Here's how the part is built. I have some questions about the finished solid (model axes, mm). A direction names the side the tool comes from. Coordinates: 2 decimals unless noted, no trailing zeros. Write each loop counter-clockwise with the first axis right and the second up, starting at its lowest first coordinate (ties: lowest second). Pieces come first, ordered by that corner, then holes.
Item 1: For faces 5 (the face through (-1.588, 200, -13)), 6 (the face through (-14.08, -18.9, -24.6)), which set-ups out of +Z, -Z, +X, -X, +Y, -Y let a thin tool reach every point of the face, with its end or its side?
Item 2: If I drill on line 1 (Y direction, x = -12.7, z = -24.8); line 2 (Z direction, x = -16.75, y = 74), over which ranges is the centre line in solid material (lowest first)?
Item 3: If we section it at A-A (z = -19.5): Please give me the cut outline in (x, y), then the cut area to 3 significant figures.
Item 4: We'd pull the mould along Y, two halves only. Please class faces 1 (the face through (-13.5, 412.7, -0.8)), 2 (the face through (-14.08, -18.9, -0.78)), 3 (the face through (-13, 200, -1.588)), 4 (the face through (-24, -25.4, -13)): +Y half, -Y half, draft (parallel to the pull), parting line (faces both ways), or undercut.
Item 5: If we section it at B-B (y = 230.5): Please give me the cut outline in (x, z).
Item 6: If we section it at C-C (x = -12.7): Count the separate pieces of the cut face and the enclosed holes in it, then the cut area to 3 significant figures.
Autodesk Inventor part; units mm, degrees
ref_plane "YZ Plane" through (0, 0, 0) normal (1, 0, 0) x (0, 1, 0)
ref_plane "XZ Plane" through (0, 0, 0) normal (0, 1, 0) x (-1, 0, 0)
ref_plane "XY Plane" through (0, 0, 0) normal (0, 0, 1) x (1, 0, 0)
sketch "Sketch1" plane through (0, 0, 0) normal (0, 1, 0) x (-1, 0, 0)
  line L0 (0, 0) -> (25.4, 0)
  line L1 (25.4, 0) -> (25.4, -25.4)
  line L2 (25.4, -25.4) -> (0, -25.4)
  line L3 (0, -25.4) -> (0, 0)
  line L4 (23.8125, -23.8125) -> (23.8125, -1.5875)
  line L5 (23.8125, -1.5875) -> (1.5875, -1.5875)
  line L6 (1.5875, -1.5875) -> (1.5875, -23.8125)
  line L7 (1.5875, -23.8125) -> (23.8125, -23.8125)
  dimension "d0" = 25.4
  dimension "d1" = 25.4
  dimension "d2" = 1.5875
extrude "Extrusion1" add sketch "Sketch1" along normal blind 419.1
sketch "Sketch3" plane through (-25.4, 0, 0) normal (0, 0, 1) x (1, 0, 0)
  point P0 (25.4, 0)
sketch "Sketch4" plane through (-25.4, 0, 0) normal (0, 0, 1) x (1, 0, 0)
  circle A0 centre (12.7, 406.4) radius 6.35
  line L0 (25.4, 0) -> (0, 0)
  line L1 (25.4, 0) -> (25.4, 419.1)
  line L2 (1.5875, 419.1) -> (23.8125, 419.1)
  dimension "d8" = 12.7
  dimension "d28" = 12.7
  dimension "d29" = 12.7
extrude "Extrusion3" cut sketch "Sketch4" against normal blind 25.4
sketch "Sketch5" plane through (-25.4, 0, 0) normal (0, 0, 1) x (1, 0, 0)
  circle A0 centre (12.7, 266.7) radius 6.35
  line L0 (25.4, 0) -> (0, 0)
  dimension "d12" = 12.7
  dimension "d15" = 266.7
extrude "Extrusion4" cut sketch "Sketch5" against normal blind 25.4
sketch "Sketch7" plane through (0, 0, 0) normal (0, -1, 0) x (1, 0, 0)
  line L0 (0, 0) -> (-25.4, 0)
  line L1 (-25.4, 0) -> (-25.4, -25.4)
  line L2 (-25.4, -25.4) -> (0, -25.4)
  line L3 (0, -25.4) -> (0, 0)
  line L4 (-1.5875, -23.8125) -> (-23.8125, -23.8125)
  line L5 (-23.8125, -1.5875) -> (-1.5875, -1.5875)
  line L6 (-23.8125, -23.8125) -> (-1.5875, -23.8125)
  line L7 (-1.5875, -23.8125) -> (-1.5875, -1.5875)
  line L8 (-1.5875, -1.5875) -> (-23.8125, -1.5875)
  line L9 (-23.8125, -1.5875) -> (-23.8125, -23.8125)
extrude "Extrusion6" add sketch "Sketch7" along normal blind 25.4
sketch "Sketch8" plane through (-25.4, 419.1, 0) normal (0, 0, 1) x (1, 0, 0)
  circle A0 centre (12.7, -431.8) radius 6.35
  line L0 (25.4, -444.5) -> (25.4, 0)
  line L1 (25.4, -444.5) -> (0, -444.5)
  point P0 (25.4, -419.1)
  dimension "d23" = 12.7
  dimension "d24" = 12.7
  dimension "d27" = 12.7
extrude "Extrusion7" cut sketch "Sketch8" against normal blind 25.4
properties part number "AP 2"
Answer list:
1. face 5: +Y, -Y
1. face 6: +Z, -Z
2. line 1: y = -25.4 to -19.05, -6.35 to 260.35, 273.05 to 400.05, 412.75 to 419.1
2. line 2: z = -25.4 to -23.81, -1.59 to 0
3. outline: (-25.4, -25.4) - (-23.81, -25.4) - (-23.81, 419.1) - (-25.4, 419.1) - close; (-1.59, -25.4) - (0, -25.4) - (0, 419.1) - (-1.59, 419.1) - close
3. area: 1,410 mm2
4. face 1: undercut
4. face 2: undercut
4. face 3: draft
4. face 4: -Y half
5. outline: (-25.4, -25.4) - (0, -25.4) - (0, 0) - (-25.4, 0) - close; hole (-23.81, -23.81) - (-1.59, -23.81) - (-1.59, -1.59) - (-23.81, -1.59) - close
6. separate pieces: 8
6. enclosed holes: 0
6. area: 1,290 mm2
